Check sheet for the drawn part. Datum: minimum x, y, z corner. Units: mm. A direction names the side the tool comes from. Coordinates: 2 decimals unless noted, no trailing zeros. Order: outer loops, then holes, each group sorted by start corner. A loop starts at its lowest first (then second) coordinate and runs counter-clockwise, first axis right, second up. Notation, with made-up numbers: (2.25, -6.75) - (8.25, -6.75) arc R19 cw to (8.25, 6.25) - close; hole circle Ø10 at (69, -34.75). An arc over 180 degrees is marked (long way). Put each result on its own line as item: value.
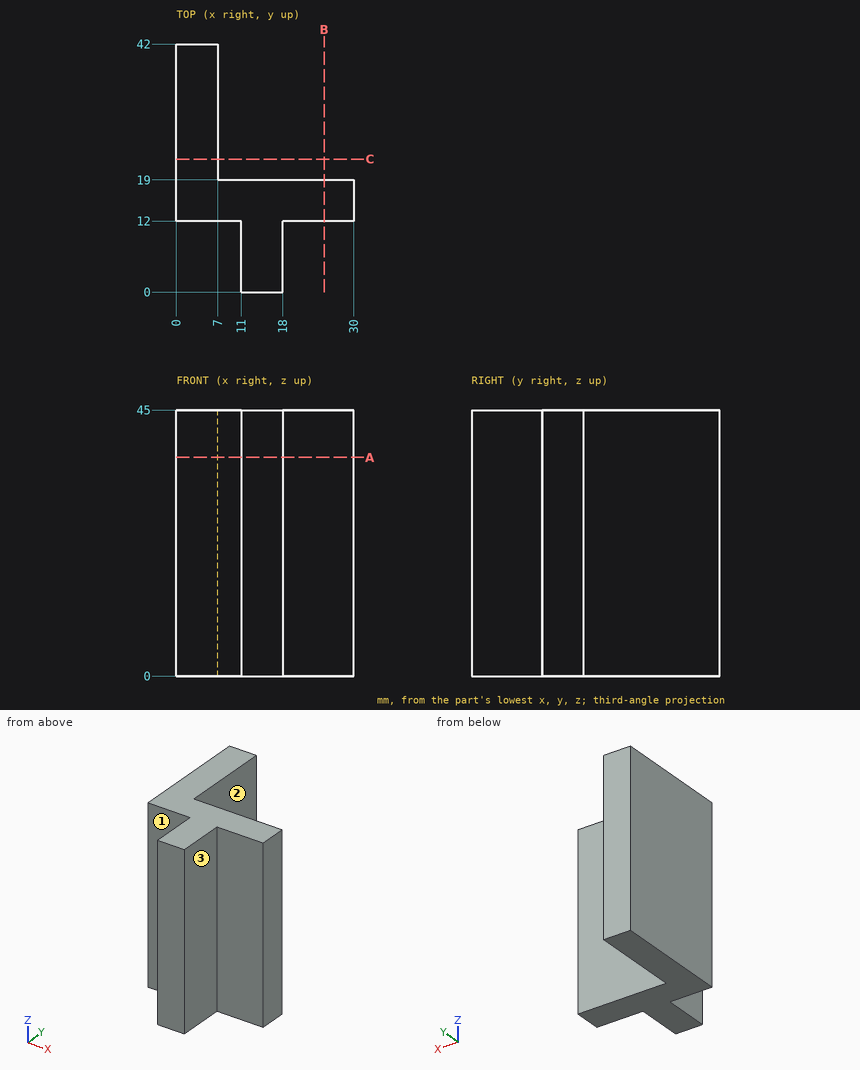
Q1. Section check A-A on z = 37. Record the boundary of the cut face in (x, y), then the cut area to 3 significant figures.
Answer block:
outline: (0, 12) - (11, 12) - (11, 0) - (18, 0) - (18, 12) - (30, 12) - (30, 19) - (7, 19) - (7, 42) - (0, 42) - close
area: 455 mm^2
Q2. Access from +Z, -Z, +X, -X, +Y, -Y to the whole of each face (thin tool, end or side, straight path). Record for the marked faces 1, 2 and 3.
Answer block:
face 1: +Z, -Z, -X, -Y
face 2: +Z, -Z, +X, +Y
face 3: +Z, -Z, +X, -Y
Q3. Depth check by flat-ended pin: pin 1 Ø3.5 at (x, z) = (21.5, 31.5) entering from -Y; pin 2 Ø6 at (y, z) = (4, 18.5) entering from +X; pin 3 Ø3.5 at (y, z) = (3.5, 16.5) entering from -X. Enter the tip coordinate at first touch or a pass-through.
Answer block:
pin 1: stops at y = 12
pin 2: stops at x = 18
pin 3: stops at x = 11
Q4. Thickness scan on L1, parallel to X at y = 2.5, z = 38.5; L2, parallel to Y at x = 8.5, z = 2; L3, parallel to X at y = 33.5, z = 41. Record the ranges inside material, lowest first. Write a range as [from, to].
Answer block:
L1: x = [11, 18]
L2: y = [12, 19]
L3: x = [0, 7]
Q5. Section check C-C on y = 22.5. Record the boundary of the cut face in (x, z).
Answer block:
outline: (0, 0) - (7, 0) - (7, 45) - (0, 45) - close
Q6. Section check B-B on x = 25. Record the boundary of the cut face in (y, z).
Answer block:
outline: (12, 0) - (19, 0) - (19, 45) - (12, 45) - close
